Verification items for the finished model (mm, model axes). Face numbers are marked on the shaded views. A direction names the side the tool comes from. Give positions to 0.01 mm unless a question says otherwise; leave off trailing zeros. Write each loop counter-clockwise with the first axis right and the second up, starting at its lowest first coordinate (ties: lowest second). Pieces come first, ordered by that corner, then holes. Notation, with made-up numbers: (23, 65.5) -> (80, 65.5) arc R13 cw to (80, 84.5) -> close; hole circle Ø7 at (-21, -39.5). An arc over 180 degrees is marked (long way). Use CSV: the item, a comma, the result in double quotes. Start each with the question number.
```python
from build123d import *

# Parameters (mm, degrees)
F0_R     = 5
F1_DEPTH = 100
F2_SIZE  = 0.5
F3_R     = 5.5
F4_DEPTH = 1


with BuildPart() as f1:
    # F0 (on Front) → F1 (new body)
    with BuildSketch(Plane.XZ):
        Circle(F0_R)
    extrude(amount=F1_DEPTH)

    # F2
    f2_edges = [f1.edges().sort_by_distance(p)[0] for p in [
        (-5, -100, 0),
    ]]
    chamfer(f2_edges, length=F2_SIZE)

    # F3 (on face) → F4 (join)
    with BuildSketch(Plane(origin=(0, 0, 0), x_dir=(-1, 0, 0), z_dir=(0, 1, 0))):
        Circle(F3_R)
    extrude(amount=-F4_DEPTH)


solid = f1.part
```
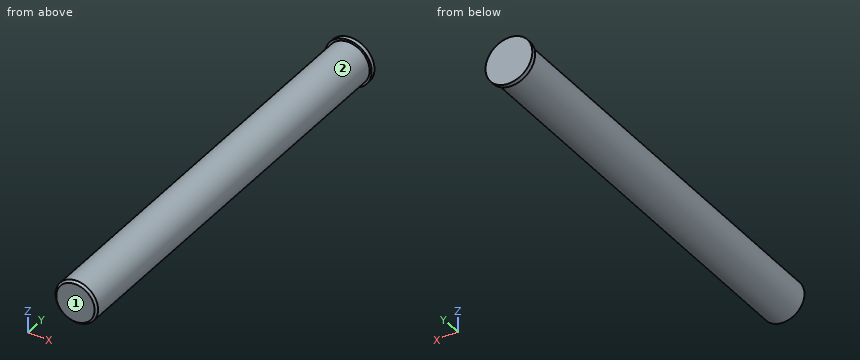
(1) Go/stop test with flat-tipped pins: pin 1 (2 mm diameter, centred on y = -79, z = -3, fed in from -X); pin 2 (6 mm diameter, centred on x = -4, y = -15.5, fed in from -Z). Record where each tip stops, or that it passes through.
(2) Thickness scan on line 1 (X direction, y = -19, z = -0.25); line 2 (X direction, y = -85, z = -4); line 3 (Z direction, x = -4.25, y = -62.5). Record the ranges inside material, lowest first. Write a range as from..to.
(3) Section check A-A on z = 0. Record the cut outline in (x, y), then the cut area to 3 significant figures.
(4) Set-up check for the marked faces 1 and 2: record each of +Z, -Z, +X, -X, +Y, -Y from which the full face is reachable in a straight line by a thin tool's end or side.
(5) Section check C-C on y = -77. Record the cut outline in (x, z), then the cut area to 3 significant figures.
(6) Section check B-B on x = 0. Record the cut outline in (y, z).
Data:
1,pin 1,"stops at x = -4.58"
1,pin 2,"stops at z = -4.9"
2,line 1,"x = -4.99..4.99"
2,line 2,"x = -3..3"
2,line 3,"z = -2.63..2.63"
3,outline,"(-5.5, -1) -> (-5, -1) -> (-5, -99.5) -> (-4.5, -100) -> (4.5, -100) -> (5, -99.5) -> (5, -1) -> (5.5, -1) -> (5.5, 0) -> (-5.5, 0) -> close"
3,area,"1,000 mm2"
4,face 1,"+Z, -Z, +X, -X, -Y"
4,face 2,"-Y"
5,outline,"circle Ø10 at (0, 0)"
5,area,"78.5 mm2"
6,outline,"(-100, -4.5) -> (-99.5, -5) -> (-1, -5) -> (-1, -5.5) -> (0, -5.5) -> (0, 5.5) -> (-1, 5.5) -> (-1, 5) -> (-99.5, 5) -> (-100, 4.5) -> close"
